Can you work these out from the model? Positions are in its coordinate system, mm. Face numbers are marked on the shaded views. A direction names the side the tool comes from. Give positions to 0.01 mm unless a question says otherwise; leave off trailing zeros. Order: outer loops, then holes, each group sorted by start corner. A loop starts at its lowest first (then second) coordinate and runs counter-clockwise, first axis right, second up. Notation, with made-up numbers: (2.5, -12.5) - (9.5, -12.5) arc R25 ccw to (9.5, 12.5) - close; hole circle Ø7 at (11, -37). An arc over 180 degrees is marked (long way). Return JSON: item names as keys, results as strings.
```python
from build123d import *

# Parameters (mm, degrees)
F_01_START                               = -1.5
S01_SOLID_POST_BLANK_16_MM_R             = 8
F_01_SOLID_POST_BLANK_16_MM_DEPTH        = 54.75
F_02_START                               = -1.6
S02_REAR_M6_HEAT_SET_INSERT_SEAT_R       = 4.05
F_02_REAR_M6_HEAT_SET_INSERT_SEAT_DEPTH  = 14.35
F_03_START                               = 39
S03_FRONT_M6_HEAT_SET_INSERT_SEAT_R      = 4.05
F_03_FRONT_M6_HEAT_SET_INSERT_SEAT_DEPTH = 14.35


with BuildPart() as part:
    # S01 - Solid post blank - 16 mm → 01 - Solid post blank - 16 mm (new body)
    with BuildSketch(Plane.XY.offset(F_01_START)):
        Circle(S01_SOLID_POST_BLANK_16_MM_R)
    extrude(amount=F_01_SOLID_POST_BLANK_16_MM_DEPTH)

    # S02 - Rear M6 heat-set insert seat → 02 - Rear M6 heat-set insert seat (cut)
    with BuildSketch(Plane.XY.offset(F_02_START)):
        Circle(S02_REAR_M6_HEAT_SET_INSERT_SEAT_R)
    extrude(amount=F_02_REAR_M6_HEAT_SET_INSERT_SEAT_DEPTH, mode=Mode.SUBTRACT)

    # S03 - Front M6 heat-set insert seat → 03 - Front M6 heat-set insert seat (cut)
    with BuildSketch(Plane.XY.offset(F_03_START)):
        Circle(S03_FRONT_M6_HEAT_SET_INSERT_SEAT_R)
    extrude(amount=F_03_FRONT_M6_HEAT_SET_INSERT_SEAT_DEPTH, mode=Mode.SUBTRACT)


solid = part.part
```
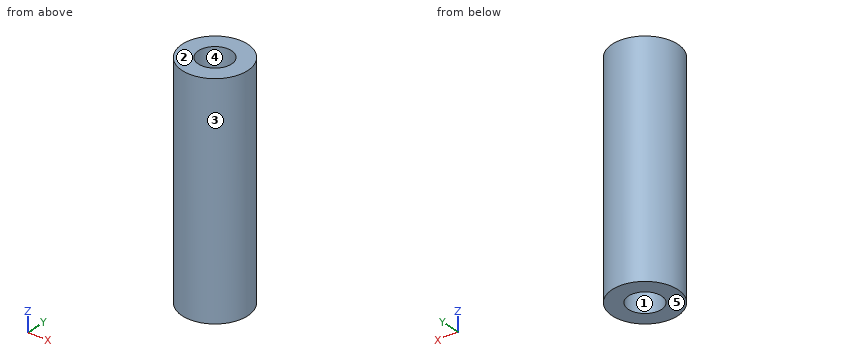
1. Suppose I cut it at D-D (x = 6). List the corners of the cut face in (y, z) for me.
Checks:
{"outline": "(-5.29, -1.5) - (5.29, -1.5) - (5.29, 53.25) - (-5.29, 53.25) - close"}
2. Thinking about a two-plate mould opening in Y: for the marked faces 3, 4 and 5, which applies, +Y half, -Y half, draft (parallel to the pull), parting line (faces both ways), or undercut?
Checks:
{"face 3": "parting line", "face 4": "undercut", "face 5": "draft"}
3. Suppose I cut it at C-C (z = 32.5). List the corners of the cut face in (x, y) for me.
Checks:
{"outline": "circle Ø16 at (0, 0)"}
4. For pin 1 Ø6.5 at (x, y) = (0, 0) entering from +Z; pin 2 Ø4 at (y, z) = (6, 14) entering from -X; pin 3 Ø1 at (x, z) = (5, 41) entering from +Y, each with a flat end and sliding along its axis, tell me the tip position at first contact or that it passes through.
Checks:
{"pin 1": "z = 39", "pin 2": "x = -6.93", "pin 3": "y = 6.61"}
5. If I drill on L1, parallel to Y at x = 0, z = 2.25; L2, parallel to Y at x = -2.5, z = 46; L3, parallel to X at y = -1, z = 41.5, over which ranges is the centre line in solid material (lowest first)? Write a range as [from, to].
Checks:
{"L1": "[-8, -4.05], [4.05, 8]", "L2": "[-7.6, -3.19], [3.19, 7.6]", "L3": "[-7.94, -3.92], [3.92, 7.94]"}
6. On a 3-axis mill with a long thin cutter (end or side, diameter ignored), from which of +Z, -Z, +X, -X, +Y, -Y can I reach the whole of each face in a straight line? I mean the marked faces 1 and 2. Say none if no direction works.
Checks:
{"face 1": "-Z", "face 2": "+Z, +X, -X, +Y, -Y"}
7. Suppose I cut it at A-A (x = 0). List the corners of the cut face in (y, z) for me, plus the area to 3 significant figures.
Checks:
{"outline": "(-8, -1.5) - (-4.05, -1.5) - (-4.05, 12.75) - (4.05, 12.75) - (4.05, -1.5) - (8, -1.5) - (8, 53.25) - (4.05, 53.25) - (4.05, 39) - (-4.05, 39) - (-4.05, 53.25) - (-8, 53.25) - close", "area": "645 mm^2"}
